```python
from build123d import *

# Parameters (mm, degrees)
CROQUIS3_W              = 2.5
CROQUIS3_H              = 93.200468797
CROQUIS3_H_2            = 93.221326365
SALIENTE_EXTRUIR1_DEPTH = 25
SALIENTE_EXTRUIR1_TAPER = 1


with BuildPart() as part:
    # Croquis1 → Revolución1 (revolve)
    with BuildSketch(Plane.XY):
        Polygon((0, 38.800633525), (0, -62.573128225), (50.821461866, -62.573128225), (50.821461866, -58.674137389), (46.92247103, -58.674137389), (46.92247103, 34.547188976), (50.821461866, 34.547188976), (50.821461866, 38.800633525), align=None)
    revolve(axis=Axis((0, 38.800633525, 0), (0, -1, 0)))

    # Croquis3 → Saliente-Extruir1 (add)
    with BuildSketch(Plane.XY):
        with Locations((-45.646866178, -12.07390299)):
            Rectangle(CROQUIS3_W, CROQUIS3_H)
        with Locations((-40.124494984, -12.063474207)):
            Rectangle(CROQUIS3_W, CROQUIS3_H_2)
    extrude(amount=-SALIENTE_EXTRUIR1_DEPTH, taper=SALIENTE_EXTRUIR1_TAPER)


solid = part.part
```
Here's how the part is built. I have some questions about the finished solid (model axes, mm). Round coordinates to 2 decimals unless told otherwise and drop trailing zeros. Order: outer loops, then holes, each group sorted by start corner. A loop starts at its lowest first (then second) coordinate and runs counter-clockwise, first axis right, second up. Notation, with made-up numbers: M 29,-7.5 L 77,-7.5 A12 cw 77,6.5 Z; hole C 84.25,44.25 d4. An arc over 180 degrees is marked long. Answer in a Markdown table with one row per item.
Item 1: Imagine slicing it at B-B, the plane z = 0. Write out the boundary of the cut face in (x, y), and give its area (3 significant figures).
A:
| item | result |
|---|---|
| outline | M -50.82,-62.57 L 50.82,-62.57 L 50.82,-58.67 L 46.92,-58.67 L 46.92,34.55 L 50.82,34.55 L 50.82,38.8 L -50.82,38.8 L -50.82,34.55 L -46.92,34.55 L -46.92,-58.67 L -50.82,-58.67 Z |
| area | 9,580 mm2 |
Item 2: If I drill on L1, parallel to X at y = -53, z = -21; L2, parallel to Z at x = -11.5, y = 1; L3, parallel to Z at x = 18, y = 27.5, over which ranges is the centre line in solid material (lowest first)? Write a range as from..to.
A:
| item | result |
|---|---|
| L1 | x = -46.53..-44.76, -41.96..41.96 |
| L2 | z = -45.49..45.49 |
| L3 | z = -43.33..43.33 |
Item 3: Imagine slicing it at A-A, the plane x = 0. Write out the boundary of the cut face in (y, z), and give its area (3 significant figures).
A:
| item | result |
|---|---|
| outline | M -62.57,-50.82 L -58.67,-50.82 L -58.67,-46.92 L 34.55,-46.92 L 34.55,-50.82 L 38.8,-50.82 L 38.8,50.82 L 34.55,50.82 L 34.55,46.92 L -58.67,46.92 L -58.67,50.82 L -62.57,50.82 Z |
| area | 9,580 mm2 |
Item 4: I'm going to push flat-ended pins straight in: pin 1 (1.4 mm diameter, centred on x = -40, y = 2, fed in from -Z); pin 2 (1.3 mm diameter, centred on x = -45.5, y = -32.5, fed in from -Z); pin 3 (8 mm diameter, centred on x = 36.5, z = 35.5, fed in from +Y); pin 4 (12 mm diameter, centred on y = 21.5, z = 12, fed in from +X). Where does each tip first touch, or does it pass through?
A:
| item | result |
|---|---|
| pin 1 | stops at z = -25.64 |
| pin 2 | stops at z = -25 |
| pin 3 | stops at y = 38.8 |
| pin 4 | stops at x = 46.54 |
Item 5: Thinking about a two-plate mould opening in Y: for faces 1 (the face through (-6.108, -11.411, 46.523)), 2 (the face through (-1, 38.801, 1)), 3 (the face through (1, -62.573, 1)), which applies, +Y half, -Y half, draft (parallel to the pull), parting line (faces both ways), or undercut?
A:
| item | result |
|---|---|
| face 1 | undercut |
| face 2 | +Y half |
| face 3 | -Y half |
